Could you check a few things on this model? Use its own coordinates, in mm. Face numbers are marked on the shaded views. A direction names the side the tool comes from. Round coordinates to 2 decimals unless told otherwise and drop trailing zeros. Loops run counter-clockwise (first coordinate to the right, second up) from the corner with the lowest first, then second, coordinate; pieces in that order, holes last. Notation, with made-up numbers: (-21.5, 38.5) - (14.5, 38.5) arc R21 cw to (14.5, 65.5) - close; hole circle Ø11 at (18, -15). An arc over 180 degrees is marked (long way). Answer as CSV lines item,"result". Start each with the question number.
1) Suppose I cut it at D-D, the plane z = 533.4. Count the separate pieces of the cut face and the enclosed holes in it, then the cut area to 3 significant figures.
2) Suppose I cut it at B-B, the plane y = 342.9. Write out the boundary of the cut face in (x, z).
3) Which directions (+Z, -Z, +X, -X, +Y, -Y) give clear straight access to the entire face, cutting with the end or side of a thin tool? Please do the marked faces 4 and 5.
4) Suppose I cut it at C-C, the plane x = -7. Write out the boundary of the cut face in (y, z) (3 decimals), then the cut area to 3 significant figures.
5) I'm going to push a flat-ended pin straight in: pin 1 Ø3 at (x, y) = (-1.5, 528.5) entering from -Z. Where does the tip first touch, or does it pass through?
6) We'd pull the mould along Y, two halves only. Please class the marked faces 1, 2 and 3: pulls with the +Y half, pulls with the -Y half, needs draft (parallel to the pull), parting line crosses it, or undercut.
7) Please list where these lines run through material, in increasing order: line 1 along Z through (x, y) = (-66, 114); line 2 along Y through (x, z) = (-0.5, 28.5) (3 decimals); line 3 along Z through (x, y) = (-17.5, 156.5).
8) Suppose I cut it at A-A, the plane z = 318. Write out the boundary of the cut face in (x, y) (3 decimals), then the cut area to 3 significant figures.
```python
from build123d import *

# Parameters (mm, degrees)
F1_DEPTH = 101.6
F2_W     = 50.8
F2_H     = 152.4
F3_DEPTH = 1581.15
F4_R     = 25.4
F5_DEPTH = 50.8


with BuildPart() as f1:
    # F0 (on Right) → F1 (new body, symmetric)
    with BuildSketch(Plane.YZ):
        Polygon((-790.575, 457.2), (-790.575, 0), (-714.375, 0), (-714.375, 381), (714.375, 381), (714.375, 0), (790.575, 0), (790.575, 457.2), align=None)
    extrude(amount=F1_DEPTH, both=True)

    # F2 (on face) → F3 (join, through all)
    with BuildSketch(Plane.XZ.offset(790.575)):
        with Locations((-76.2, 533.4)):
            Rectangle(F2_W, F2_H)
    extrude(amount=-F3_DEPTH)

    # F4 (on face) → F5 (cut, through all)
    with BuildSketch(Plane.YZ.offset(-50.8)):
        with Locations((-457.2, 533.4)):
            Circle(F4_R)
        with Locations((-342.9, 533.4)):
            Circle(F4_R)
        with Locations((-228.6, 533.4)):
            Circle(F4_R)
        with Locations((-114.3, 533.4)):
            Circle(F4_R)
        with Locations((0, 533.4)):
            Circle(F4_R)
        with Locations((-685.8, 533.4)):
            Circle(F4_R)
        with Locations((-571.5, 533.4)):
            Circle(F4_R)
        with Locations((114.3, 533.4)):
            Circle(F4_R)
        with Locations((228.6, 533.4)):
            Circle(F4_R)
        with Locations((342.9, 533.4)):
            Circle(F4_R)
        with Locations((457.2, 533.4)):
            Circle(F4_R)
        with Locations((571.5, 533.4)):
            Circle(F4_R)
        with Locations((685.8, 533.4)):
            Circle(F4_R)
    extrude(amount=-F5_DEPTH, mode=Mode.SUBTRACT)


solid = f1.part
```
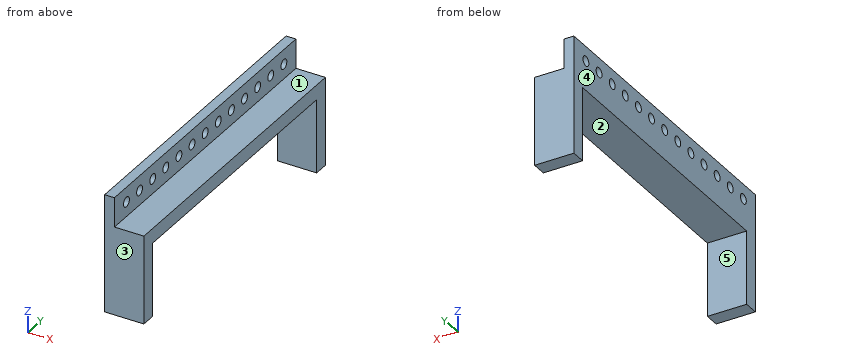
Filled sheet:
1,separate pieces,"14"
1,enclosed holes,"0"
1,area,"46,800 mm²"
2,outline,"(-101.6, 381) - (101.6, 381) - (101.6, 457.2) - (-50.8, 457.2) - (-50.8, 508) - (-101.6, 508) - close; (-101.6, 558.8) - (-50.8, 558.8) - (-50.8, 609.6) - (-101.6, 609.6) - close"
3,face 4,"+Z, -Z, -X, +Y, -Y"
3,face 5,"-Z, +X, -X"
4,outline,"(-790.575, 0) - (-714.375, 0) - (-714.375, 381) - (714.375, 381) - (714.375, 0) - (790.575, 0) - (790.575, 457.2) - (-790.575, 457.2) - close"
4,area,"179,000 mm²"
5,pin 1,"z = 381"
6,face 1,"needs draft"
6,face 2,"undercut"
6,face 3,"pulls with the -Y half"
7,line 1,"381 to 508, 558.8 to 609.6"
7,line 2,"-790.575 to -714.375, 714.375 to 790.575"
7,line 3,"381 to 457.2"
8,outline,"(-101.6, -790.575) - (101.6, -790.575) - (101.6, -714.375) - (-101.6, -714.375) - close; (-101.6, 714.375) - (101.6, 714.375) - (101.6, 790.575) - (-101.6, 790.575) - close"
8,area,"31,000 mm²"
